Read the model definition and answer for the solid it produces. Units are mm, in the model's axes. A direction names the side the tool comes from. Coordinates: 2 decimals unless noted, no trailing zeros. Order: outer loops, then holes, each group sorted by start corner. A loop starts at its lowest first (then second) coordinate and runs counter-clockwise, first axis right, second up. Notation, with made-up numbers: M 52.5,56.25 L 102.5,56.25 A12 cw 102.5,71.25 Z; hole C 12.5,-21 d8. An arc over 180 degrees is marked long. One line per question, with ' | ' between items. Start each with the question number.
1) The mould has two halves that part along X. Classify faces 1 (the face through (0, 6, 3)), 2 (the face through (-7, 25, -8)), 3 (the face through (-6.94, -31.24, 5.09)): +X half, -X half, draft (parallel to the pull), parting line (faces both ways), or undercut.
2) Find section D-D, the plane z = 10.75. Write down the section's boundary in (x, y).
3) Consider probe 1 along Y at (x, z) = (0, 6); probe 2 along Y at (x, z) = (-20.5, 9.75); probe 3 along Z at (x, y) = (-22.5, -20). Determine where each line is inside the solid, lowest interval first.
4) Find section A-A, the plane x = 0. Write down the section's boundary in (y, z), plus the area to 3 significant figures.
5) A tool of negligible diameter and unlimited length cuts with its end or side. For faces 4 (the face through (-5.172, 3.042, 2.972)), 5 (the face through (-7, 25, 18.5)), 6 (the face through (0, -5, 7.5)), from which of +Z, -Z, +X, -X, +Y, -Y can it reach the whole face along a straight path? Write none if from no direction.
6) Find section C-C, the plane z = 6.25. Write down the section's boundary in (x, y).
7) Find section B-B, the plane z = 2.25. Write down the section's boundary in (x, y), plus the area to 3 significant figures.
8) Given P1, Ø6, axis at x = 4, y = 3.5, coming from the +Z side; P2, Ø10, axis at y = 23, z = 12.5, coming from the +X side; P3, Ø5, axis at x = 0, y = 0, coming from the -Z side, each flat-ended and moving along its own axis, determine where each tip first touches the part or whether it passes through.
from build123d import *

# Parameters (mm, degrees)
EXTRUDE_START   = 1
SKETCH_1_R      = 25
EXTRUDE_1_DEPTH = 4
SKETCH_4_R      = 25
SKETCH_4_R_2    = 2
EXTRUDE_3_DEPTH = 2.5
EXTRUDE_START_2 = -15.5
SKETCH_6_R      = 32
SKETCH_6_R_2    = 25
EXTRUDE_4_DEPTH = 26.5
FILLET_1_R      = 2


with BuildPart() as part:
    # 草图1 → 凸台-拉伸1 (new body)
    with BuildSketch(Plane.XY.offset(EXTRUDE_START)):
        Circle(SKETCH_1_R)
        Polygon((3.464101615, 6), (-3.464101615, 6), (-6.92820323, 0), (-3.464101615, -6), (3.464101615, -6), (6.92820323, 0), align=None, mode=Mode.SUBTRACT)
    extrude(amount=EXTRUDE_1_DEPTH)

    # 草图4 → 凸台-拉伸3 (add)
    with BuildSketch(Plane.XY.offset(5)):
        Circle(SKETCH_4_R)
        Circle(SKETCH_4_R_2, mode=Mode.SUBTRACT)
    extrude(amount=EXTRUDE_3_DEPTH)

    # 草图6 → 凸台-拉伸4 (add)
    with BuildSketch(Plane.XY.offset(7.5).offset(EXTRUDE_START_2)):
        Circle(SKETCH_6_R)
        Circle(SKETCH_6_R_2, mode=Mode.SUBTRACT)
    extrude(amount=EXTRUDE_4_DEPTH)

    # 圆角1
    fillet_1_edges = [part.edges().sort_by_distance(p)[0] for p in [
        (-32, 0, -8),
        (-32, 0, 18.5),
    ]]
    fillet(fillet_1_edges, radius=FILLET_1_R)


solid = part.part
Report:
1) face 1: undercut | face 2: draft | face 3: parting line
2) outline: C 0,0 d64; hole C 0,0 d50
3) probe 1: y = -32 to -2, 2 to 32 | probe 2: y = -24.57 to -14.31, 14.31 to 24.57 | probe 3: z = -8 to 18.5
4) outline: M -32,-6 A2 ccw -30,-8 L -25,-8 L -25,1 L -6,1 L -6,5 L -2,5 L -2,7.5 L -25,7.5 L -25,18.5 L -30,18.5 A2 ccw -32,16.5 Z; M 2,5 L 6,5 L 6,1 L 25,1 L 25,-8 L 30,-8 A2 ccw 32,-6 L 32,16.5 A2 ccw 30,18.5 L 25,18.5 L 25,7.5 L 2,7.5 Z | area: 635 mm^2
5) face 4: -Z | face 5: +Z, +X, -X, +Y, -Y | face 6: +Z
6) outline: C 0,0 d64; hole C 0,0 d4
7) outline: C 0,0 d64; hole M -6.93,0 L -3.46,-6 L 3.46,-6 L 6.93,0 L 3.46,6 L -3.46,6 Z | area: 3,090 mm^2
8) P1: stops at z = 7.5 | P2: stops at x = 26.46 | P3: stops at z = 5
